Work out the finished part from the listing and answer in its coordinate system (mm). A direction names the side the tool comes from. Round coordinates to 2 decimals unless told otherwise and drop trailing zeros. Order: outer loops, then holes, each group sorted by start corner. A loop starts at its lowest first (then second) coordinate and runs counter-clockwise, first axis right, second up. Notation, with made-up numbers: (73, -24) - (123, -24) arc R20 ccw to (123, -12) - close; hole circle Ø3 at (-8.75, -21). An arc over 180 degrees is marked (long way). Put each result on its own line as item: value.
Autodesk Inventor part; units mm, degrees
ref_plane "YZ Plane" through (0, 0, 0) normal (1, 0, 0) x (0, 1, 0)
ref_plane "XZ Plane" through (0, 0, 0) normal (0, 1, 0) x (-1, 0, 0)
ref_plane "XY Plane" through (0, 0, 0) normal (0, 0, 1) x (1, 0, 0)
sketch "Sketch1" plane through (0, 0, 0) normal (1, 0, 0) x (0, 1, 0)
  line L0 (76.2, 254) -> (-76.2, 254)
  line L1 (-76.2, 254) -> (-76.2, -254)
  line L2 (-76.2, -254) -> (76.2, -254)
  line L3 (76.2, -254) -> (76.2, 254)
  line L4 (76.2, 254) -> (-76.2, -254) construction
  line L5 (-76.2, 254) -> (76.2, -254) construction
  line L6 (50.8, 279.4) -> (-50.8, 279.4)
  line L7 (-50.8, 279.4) -> (-50.8, 254)
  line L8 (-50.8, 254) -> (50.8, 254)
  line L9 (50.8, 254) -> (50.8, 279.4)
  line L10 (50.8, 279.4) -> (-50.8, 254) construction
  line L11 (-50.8, 279.4) -> (50.8, 254) construction
  line L12 (50.8, -254) -> (-50.8, -254)
  line L13 (-50.8, -254) -> (-50.8, -279.4)
  line L14 (-50.8, -279.4) -> (50.8, -279.4)
  line L15 (50.8, -279.4) -> (50.8, -254)
  line L16 (50.8, -254) -> (-50.8, -279.4) construction
  line L17 (-50.8, -254) -> (50.8, -279.4) construction
  line L18 (0, 266.7) -> (0, -266.7) construction
  point P0 (0, 0)
  point P1 (-50.8, -254)
  point P2 (50.8, 254)
  dimension "d0" = 152.4
  dimension "d1" = 508
  dimension "d9" = 25.4
  dimension "d10" = 101.6
extrude "Extrusion1" add sketch "Sketch1" along normal mid plane 6.35
sketch "Sketch3" plane through (3.175, 0, 0) normal (1, 0, 0) x (0, 0, -1)
  line L0 (-241.3, 44.45) -> (-201.6125, 44.45)
  line L1 (-201.6125, 44.45) -> (-201.6125, -44.45)
  line L2 (-201.6125, -44.45) -> (-241.3, -44.45)
  line L3 (-241.3, -44.45) -> (-241.3, 44.45)
  line L4 (-179.3875, 44.45) -> (-125.857, 44.45)
  line L5 (-125.857, 44.45) -> (-125.857, -44.45)
  line L6 (-125.857, -44.45) -> (-179.3875, -44.45)
  line L7 (-179.3875, -44.45) -> (-179.3875, 44.45)
  line L8 (-103.632, 44.45) -> (50.8, 44.45)
  line L9 (50.8, 44.45) -> (50.8, -44.45)
  line L10 (50.8, -44.45) -> (-103.632, -44.45)
  line L11 (-103.632, -44.45) -> (-103.632, 44.45)
  line L12 (74.6125, 44.45) -> (179.3875, 44.45)
  line L13 (179.3875, 44.45) -> (179.3875, -44.45)
  line L14 (179.3875, -44.45) -> (74.6125, -44.45)
  line L15 (74.6125, -44.45) -> (74.6125, 44.45)
  line L16 (201.6125, -44.45) -> (241.3, -44.45)
  line L17 (241.3, -44.45) -> (241.3, 44.45)
  line L18 (241.3, 44.45) -> (201.6125, 44.45)
  line L19 (201.6125, 44.45) -> (201.6125, -44.45)
  line L20 (-201.6125, 0) -> (-179.3875, 0) construction
  line L21 (-125.857, 0) -> (-103.632, 0) construction
  line L22 (179.3875, 0) -> (201.6125, 0) construction
  line L23 (-254, -50.8) -> (-254, -76.2) construction
  circle A0 centre (-190.5, 63.5) radius 3.175
  line L24 (-190.5, 63.5) -> (-190.5, 0) construction
  line L25 (-190.5, 0) -> (-190.5, -63.5) construction
  circle A1 centre (-190.5, -63.5) radius 3.9751
  circle A2 centre (-63.5, 63.5) radius 3.175
  circle A3 centre (-63.5, -63.5) radius 3.9751
  circle A4 centre (63.5, 63.5) radius 3.175
  circle A5 centre (63.5, -63.5) radius 3.9751
  circle A6 centre (190.5, 63.5) radius 3.175
  circle A7 centre (190.5, -63.5) radius 3.9751
  line L26 (-125.857, 44.45) -> (-103.632, 44.45)
  line L27 (-103.632, 44.45) -> (-103.632, -44.45)
  line L28 (-103.632, -44.45) -> (-125.857, -44.45)
  line L29 (-125.857, -44.45) -> (-125.857, 44.45)
  line L30 (254, -76.2) -> (254, -50.8)
  line L31 (-254, -76.2) -> (254, -76.2)
  point P0 (0, 0)
  point P1 (0, 0)
  point P2 (-114.7445, 0)
  dimension "d12" = 22.225
  dimension "d13" = 12.7
  dimension "d14" = 88.9
  dimension "d16" = 6.35
  dimension "d17" = 7.9502
  dimension "d20" = 127
  dimension "d29" = 12.7
  dimension "d30" = 63.5
  dimension "d31" = 12.7
  dimension "d32" = 11.1125
  dimension "d33" = 31.75
  dimension "d34" = 127
  dimension "d35" = 63.5
  dimension "d39" = 154.432
extrude "Extrusion3" cut sketch "Sketch3" against normal through all contours L0 L1 L2 L3 | L4 L5 L6 L7 | L8 L9 L10 L11 | L12 L13 L14 L15 | L19 L18 L17 L16 | A0 | A1 | A2 | A3 | A4 | A5 | A6 | A7
fillet "Fillet1" radius 12.7 24 edges at (0, 50.8, 279.4) (0, 44.45, 241.3) (0, 44.45, 201.6125) (0, -44.45, 201.6125) (0, -44.45, 241.3) (0, -50.8, 279.4) (0, -44.45, 179.3875) (0, 44.45, 179.3875) (0, -44.45, -50.8) (0, -44.45, -74.6125) (0, 44.45, -74.6125) (0, 44.45, -50.8) (0, 44.45, -179.3875) (0, 44.45, -201.6125) (0, 44.45, -241.3) (0, 50.8, -279.4) (0, -50.8, -279.4) (0, -44.45, -241.3) (0, -44.45, -201.6125) (0, -44.45, -179.3875) (0, 44.45, 125.857) (0, 44.45, 103.632) (0, -44.45, 103.632) (0, -44.45, 125.857)
fillet "Fillet1" radius 1.5875 8 edges at (0, 50.8, 254) (0, -50.8, 254) (0, -76.2, 254) (0, 76.2, 254) (0, 76.2, -254) (0, 50.8, -254) (0, -50.8, -254) (0, -76.2, -254)
sketch "Sketch4" plane through (-3.175, 0, 0) normal (-1, 0, 0) x (0, 0, 1)
  line L0 (-182.626, 63.5635) -> (-141.351, 63.5635) construction
  line L1 (-254, 74.6125) -> (-254, 52.3875) construction
  line L2 (252.4125, 76.2) -> (-252.4125, 76.2) construction
  point P0 (0, 0)
  dimension "d36" = 71.374
  dimension "d37" = 12.6365
  dimension "d38" = 41.275
properties part number "ChassisInterface" material "Aluminum 6061"
1) Straight lines are drawn through the part: L1, parallel to Y at x = 0.75, z = -190.5 (3 decimals); L2, parallel to Z at x = -0.25, y = 28.5; L3, parallel to Y at x = -1.25, z = -87. For each, find the intervals that lie inside material, in ascending order. Write a range as from..to.
Findings below:
L1: y = -76.2..-67.475, -59.525..60.325, 66.675..76.2
L2: z = -279.4..-241.3, -201.61..-179.39, -74.61..-50.8, 103.63..125.86, 179.39..201.61, 241.3..279.4
L3: y = -76.2..-44.45, 44.45..76.2
2) For a pull along Z with two mould halves and no side action, classify faces 3 (the cylindrical face through (0.04, -46.98, 275.78)), 4 (the cylindrical face through (-0.044, 40.631, 175.766)), 5 (the cylindrical face through (-0.044, 40.631, -78.234)), 6 (the flat face through (-3.175, 50, 4)) as pulls with the +Z half, pulls with the -Z half, needs draft (parallel to the pull), parting line crosses it, or undercut.
Findings below:
face 3: pulls with the +Z half
face 4: undercut
face 5: undercut
face 6: needs draft
3) Given pin 1 Ø1.9 at (x, z) = (-0.5, -263.5) entering from -Y; pin 2 Ø1.9 at (x, z) = (1, 260.5) entering from +Y; pin 3 Ø5 at (y, z) = (-63.5, 190.5) entering from -X; pin 4 Ø3 at (x, y) = (-1, 65) entering from +Z, each flat-ended and moving along its own axis, determine where each tip first touches the part or whether it passes through.
Findings below:
pin 1: stops at y = -50.8
pin 2: stops at y = 50.8
pin 3: passes through
pin 4: stops at z = 254
4) For faces 1 (the cylindrical face through (0.04, -47.18, -275.58)), 2 (the cylindrical face through (-0.04, -40.63, 129.48)), determine the directions among +Z, -Z, +X, -X, +Y, -Y from which every point of the face is accessible in a straight line to the end or side of a thin tool.
Findings below:
face 1: -Z, +X, -X, -Y
face 2: +X, -X
5) A cutting plane is placed at A-A on z = -97. Write down the section's boundary in (x, y) (3 decimals).
Findings below:
outline: (-3.175, -76.2) - (3.175, -76.2) - (3.175, -44.45) - (-3.175, -44.45) - close; (-3.175, 44.45) - (3.175, 44.45) - (3.175, 76.2) - (-3.175, 76.2) - close
6) A cutting plane is placed at B-B on y = -18.5. Write down the section's boundary in (x, z) (1 decimal).
Findings below:
outline: (-3.2, -279.4) - (3.2, -279.4) - (3.2, -241.3) - (-3.2, -241.3) - close; (-3.2, -201.6) - (3.2, -201.6) - (3.2, -179.4) - (-3.2, -179.4) - close; (-3.2, -74.6) - (3.2, -74.6) - (3.2, -50.8) - (-3.2, -50.8) - close; (-3.2, 103.6) - (3.2, 103.6) - (3.2, 125.9) - (-3.2, 125.9) - close; (-3.2, 179.4) - (3.2, 179.4) - (3.2, 201.6) - (-3.2, 201.6) - close; (-3.2, 241.3) - (3.2, 241.3) - (3.2, 279.4) - (-3.2, 279.4) - close
7) A cutting plane is placed at C-C on x = -1.5. Give the number of separate pieces and of enclosed holes in the cut face, then the cut area to 3 significant figures.
Findings below:
separate pieces: 1
enclosed holes: 13
area: 48,000 mm2
